Source: three-view drawing plus pictorial views. Frame: mm from the lowest corner of the part. A direction names the side the tool comes from. Give positions to 0.01 mm unless a question says otherwise; leave off trailing zeros. Loops run counter-clockwise (first coordinate to the right, second up) from the corner with the lowest first, then second, coordinate; pieces in that order, holes last. Notation, with made-up numbers: (-29.75, 85) - (-5.75, 85) arc R18 cw to (-5.75, 114) - close; hole circle Ø9 at (70, -16). An arc over 180 degrees is marked (long way). Answer as a JSON object with one key per item and string values.
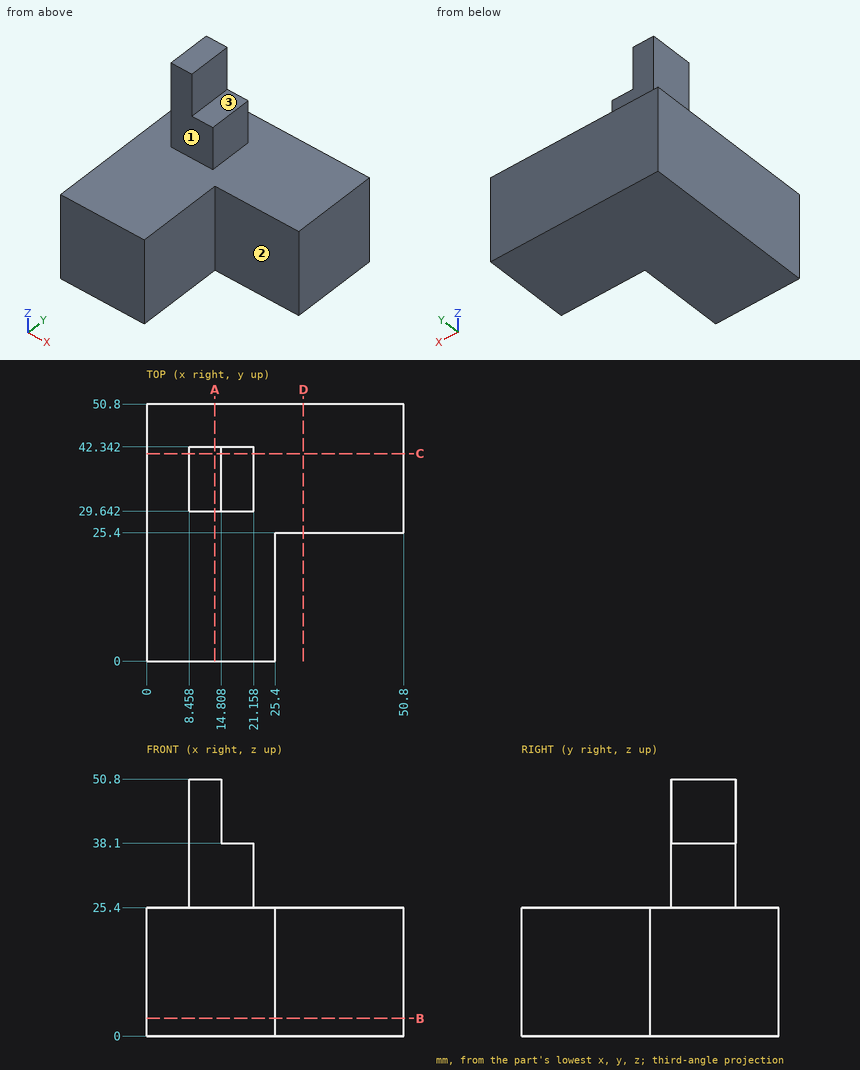
Item 1: Material intervals for line 1 (Z direction, x = 22, y = 42); line 2 (X direction, y = 36.5, z = 31.5), sorted ascending. Write a range as [from, to].
Geometry check:
{"line 1": "z = [0, 25.4]", "line 2": "x = [8.46, 21.16]"}
Item 2: Access query for the marked faces 1, 2 and 3. Directions: +Z, -Z, +X, -X, +Y, -Y. A direction counts if a zero-diameter tool reaches every point of the face in a straight line with its end or side. Return the directions, or none.
Geometry check:
{"face 1": "+Z, +X, -X, -Y", "face 2": "+Z, -Z, +X, -Y", "face 3": "+Z, +X, +Y, -Y"}
Item 3: Contact query for flat-ended pins moving along their axis: P1, Ø4, axis at y = 34, z = 47, coming from the +X side; P2, Ø7.5, axis at x = 34, z = 14, coming from the -Y side; P3, Ø14, axis at x = 15.5, z = 35.5, coming from the +Y side. Output: stop coordinate, or through.
Geometry check:
{"P1": "stops at x = 14.81", "P2": "stops at y = 25.4", "P3": "stops at y = 42.34"}
Item 4: Cut plane B-B (z = 3.5). Return loops of the section in (x, y), then the cut area to 3 significant figures.
Geometry check:
{"outline": "(0, 0) - (25.4, 0) - (25.4, 25.4) - (50.8, 25.4) - (50.8, 50.8) - (0, 50.8) - close", "area": "1,940 mm2"}
Item 5: Cut plane C-C (y = 41). Return loops of the section in (x, z), then the cut area to 3 significant figures.
Geometry check:
{"outline": "(0, 0) - (50.8, 0) - (50.8, 25.4) - (21.16, 25.4) - (21.16, 38.1) - (14.81, 38.1) - (14.81, 50.8) - (8.46, 50.8) - (8.46, 25.4) - (0, 25.4) - close", "area": "1,530 mm2"}
Item 6: Cut plane A-A (x = 13.5). Return loops of the section in (y, z), then the cut area to 3 significant figures.
Geometry check:
{"outline": "(0, 0) - (50.8, 0) - (50.8, 25.4) - (42.34, 25.4) - (42.34, 50.8) - (29.64, 50.8) - (29.64, 25.4) - (0, 25.4) - close", "area": "1,610 mm2"}
Item 7: Cut plane D-D (x = 31). Return loops of the section in (y, z), then the cut area to 3 significant figures.
Geometry check:
{"outline": "(25.4, 0) - (50.8, 0) - (50.8, 25.4) - (25.4, 25.4) - close", "area": "645 mm2"}
